Autodesk Fusion 360 part; units mm, degrees
box "BoxPrimitive1" add length 120 width 30 height 35 placed x (0, 0, -1) y (-1, 0, 0) z (0, 1, 0) at (30, 0, 0)
sketch "Sketch2" plane through (0, 0, 0) normal (0, 0, 1) x (1, 0, 0)
  line L0 (0, 35) -> (0, 0)
  line L1 (0, 0) -> (30, 0)
  line L2 (30, 0) -> (30, 35)
  line L3 (30, 35) -> (0, 35)
  line L4 (15, 0) -> (23, 0)
  line L5 (15, 0) -> (7, 0)
  line L6 (15, 0) -> (15, 10) construction
  line L7 (15, 10) -> (7, 0)
  line L8 (15, 10) -> (23, 0)
  dimension "d6" = 8
  dimension "d7" = 8
  dimension "d8" = 10
extrude "Extrude1" cut sketch "Sketch2" against normal blind 180.216 contours L1 L4 L5 L7 L8
sketch "Sketch3" plane through (30, 0, 0) normal (1, 0, 0) x (0, 0, -1)
  line L0 (0, 35) -> (0, 0)
  line L1 (0, 0) -> (120, 0)
  line L2 (120, 0) -> (120, 35)
  line L3 (120, 35) -> (0, 35)
  line L4 (0, 0) -> (25, 0)
  line L5 (120, 0) -> (95, 0)
  arc A0 (95, 0) -> (25, 0) centre (60, -20.625) ccw
  dimension "d11" = 25
  dimension "d12" = 25
extrude "Extrude2" cut sketch "Sketch3" against normal blind 49.649 contours L1 A0
sketch "Sketch4" plane through (0, 35, 0) normal (0, 1, 0) x (-1, 0, 0)
  line L0 (-30, -120) -> (0, -120)
  line L1 (0, -120) -> (0, 0)
  line L2 (0, 0) -> (-30, 0)
  line L3 (-30, 0) -> (-30, -120)
  line L4 (-30, 0) -> (-30, -10)
  line L5 (-30, -120) -> (-30, -110)
  line L6 (-30, -10) -> (0, -10)
  line L7 (0, -10) -> (0, -14)
  line L8 (0, -14) -> (-30, -14)
  line L9 (-30, -14) -> (-30, -10)
  line L10 (-30, -110) -> (0, -110)
  line L11 (0, -110) -> (0, -106)
  line L12 (0, -106) -> (-30, -106)
  line L13 (-30, -106) -> (-30, -110)
  dimension "d15" = 10
  dimension "d16" = 10
  dimension "d17" = 4
  dimension "d18" = 4
extrude "Extrude3" cut sketch "Sketch4" against normal blind 3 contours L1 L3 L6 L7 L8 L9
extrude "Extrude4" cut sketch "Sketch4" against normal blind 3 contours L1 L3 L10 L11 L12 L13
move_face "OffsetFaces1" offset -1 1 faces at (10, 33, -14)
move_face "OffsetFaces2" offset -1 1 faces at (10, 33, -106)
fillet "Fillet1" radius 1 1 edges at (30, 35, -60)
fillet "Fillet2" radius 1 3 edges at (30, 33, -105) (29.7071, 34.7071, -105) (14.5, 35, -105)
fillet "Fillet3" radius 1 1 edges at (30, 35, -115)
fillet "Fillet4" radius 1 3 edges at (30, 17, -120) (29.7071, 34.7071, -120) (14.5, 35, -120)
fillet "Fillet5" radius 1 3 edges at (0, 17, -120) (0, 34.7071, -119.7071) (0, 35, -114.5)
fillet "Fillet6" radius 1 5 edges at (0, 33, -110) (0.2929, 34.7071, -110) (15, 35, -110) (29.7071, 34.7071, -110) (30, 33, -110)
fillet "Fillet7" radius 1 3 edges at (0, 33, -105) (0, 34.7071, -104.7071) (0, 35, -59.5)
fillet "Fillet8" radius 1 5 edges at (0, 33, -15) (0.2929, 34.7071, -15) (15, 35, -15) (29.7071, 34.7071, -15) (30, 33, -15)
fillet "Fillet9" radius 1 1 edges at (30, 33.5, -10)
fillet "Fillet10" radius 1 1 edges at (0, 33.5, -10)
fillet "Fillet11" radius 1 5 edges at (30, 35, -4.5) (29.7071, 35, -9.7071) (15, 35, -10) (0.2929, 35, -9.7071) (0, 35, -4.5)
fillet "Fillet12" radius 1 5 edges at (0, 17, 0) (0.2929, 34.7071, 0) (15, 35, 0) (29.7071, 34.7071, 0) (30, 17, 0)
fillet "Fillet13" radius 1 1 edges at (30, 20, -60)
fillet "Fillet14" radius 1 1 edges at (0, 20, -60)
fillet "Fillet15" radius 3 1 edges at (23, 0, -12.5)
fillet "Fillet16" radius 3 1 edges at (7, 0, -12.5)
fillet "Fillet17" radius 3 1 edges at (23, 0, -107.5)
fillet "Fillet18" radius 3 1 edges at (7, 0, -107.5)
Check sheet for the modelled part. Datum: model origin and axes. Units: mm. A direction names the side the tool comes from. Round coordinates to 2 decimals unless told otherwise and drop trailing zeros. Order: outer loops, then holes, each group sorted by start corner. A loop starts at its lowest first (then second) coordinate and runs counter-clockwise, first axis right, second up.
Q1. Cross-section at A-A, the plane z = -102. Enter the section's corners in (x, y), plus the area to 3 significant figures.
Filled sheet:
outline: (0, 0) - (5.56, 0) arc R3 ccw to (7.9, 1.13) - (15, 10) - (22.1, 1.13) arc R3 ccw to (24.44, 0) - (30, 0) - (30, 34) arc R1 ccw to (29, 35) - (1, 35) arc R1 ccw to (0, 34) - close
area: 969 mm2
Q2. Draft check along X on faces 4 (the face through (30, 24, -61)), 5 (the face through (15, 17, 0)), 6 (the face through (6.841, 0.288, -12.664)). Enter one of: pulls with the +X half, pulls with the -X half, needs draft (parallel to the pull), parting line crosses it, or undercut.
Filled sheet:
face 4: pulls with the +X half
face 5: needs draft
face 6: undercut
Q3. Cross-section at C-C, the plane y = 4. Give the number of separate pieces and of enclosed holes in the cut face, plus the area to 3 significant figures.
Filled sheet:
separate pieces: 4
enclosed holes: 0
area: 1,130 mm2
Q4. Set-up check for faces 1 (the face through (15, 33, -105)), 2 (the face through (27, 0, -107)), 3 (the face through (6.841, 0.288, -106.976)): record each of +Z, -Z, +X, -X, +Y, -Y from which the full face is reachable in a straight line by a thin tool's end or side.
Filled sheet:
face 1: +X, -X, +Y
face 2: +Z, -Z, +X, -X, -Y
face 3: +Z, -Z, -Y
Q5. Scan lines: L1, parallel to Z at x = 25.5, y = 32.5; L2, parallel to X at y = 9, z = -27; L3, parallel to Z at x = 3.5, y = 8. Record each from-to range of solid material in increasing order.
Filled sheet:
L1: z = -120 to -110, -105 to -15, -10 to 0
L2: x = 0 to 14.2, 15.8 to 30
L3: z = -120 to -88.83, -31.17 to 0
Q6. Depth check by flat-ended pin: P1, Ø3, axis at y = 16.5, z = -66.5, coming from the -X side; P2, Ø4, axis at x = 22, z = -71.5, coming from the -Y side; P3, Ø3.5, axis at x = 14, z = -12.5, coming from the +Y side. Enter the tip coordinate at first touch or a pass-through.
Filled sheet:
P1: passes through
P2: stops at y = 17.69
P3: stops at y = 32
Q7. Cross-section at B-B, the plane x = 10.5. Enter the section's corners in (y, z) (3 decimals), plus the area to 3 significant figures.
Filled sheet:
outline: (4.375, -120) - (34, -120) arc R1 ccw to (35, -119) - (35, -111) arc R1 ccw to (34, -110) - (32, -110) - (32, -105) - (34, -105) arc R1 ccw to (35, -104) - (35, -16) arc R1 ccw to (34, -15) - (32, -15) - (32, -10) - (34, -10) arc R1 ccw to (35, -9) - (35, -1) arc R1 ccw to (34, 0) - (4.375, 0) - (4.375, -27.978) arc R40.625 cw to (4.375, -92.022) - close
area: 2,950 mm2
